```python
from build123d import *

# Parameters (mm, degrees)
EXTRUDE_1_DEPTH = 3


with BuildPart() as part:
    # 草圖1 → 填料-伸長1 (new body)
    with BuildSketch(Plane.XY):
        with BuildLine():
            Line((-282, -10), (-10, -10))
            Line((-10, -10), (-10, -3))
            ThreePointArc((-10, -3), (-9.121320344, -0.878679656), (-7, 0))
            Line((-7, 0), (7, 0))
            ThreePointArc((7, 0), (9.121320344, -0.878679656), (10, -3))
            Line((10, -3), (10, -10))
            Line((10, -10), (282, -10))
            Line((282, -10), (282, 10))
            Line((282, 10), (-282, 10))
            Line((-282, 10), (-282, -10))
        make_face()
    extrude(amount=EXTRUDE_1_DEPTH)


solid = part.part
```
Design review of the part built by this model. Coordinates are the model's own, in mm. Coordinates: 2 decimals unless noted, no trailing zeros. Loops run counter-clockwise (first coordinate to the right, second up) from the corner with the lowest first, then second, coordinate; pieces in that order, holes last.
Q1. We need section B-B on z = 0.45. State the section outline as (x, y) points, and give its area (3 significant figures).
Reported:
outline: (-282, -10) - (-10, -10) - (-10, -3) arc R3 cw to (-7, 0) - (7, 0) arc R3 cw to (10, -3) - (10, -10) - (282, -10) - (282, 10) - (-282, 10) - close
area: 11,100 mm2
Q2. We need section A-A on y = -6.5. State the section outline as (x, z) points.
Reported:
outline: (-282, 0) - (-10, 0) - (-10, 3) - (-282, 3) - close; (10, 0) - (282, 0) - (282, 3) - (10, 3) - close
Q3. To check wall thickness, follow line 1 (X direction, y = -8.75, z = 1.85); line 2 (X direction, y = -1.75, z = 0.8); line 3 (Y direction, x = -9, z = 2.6). State the ranges of each line that lie inside material, in increasing order.
Reported:
line 1: x = -282 to -10, 10 to 282
line 2: x = -282 to -9.73, 9.73 to 282
line 3: y = -0.76 to 10
